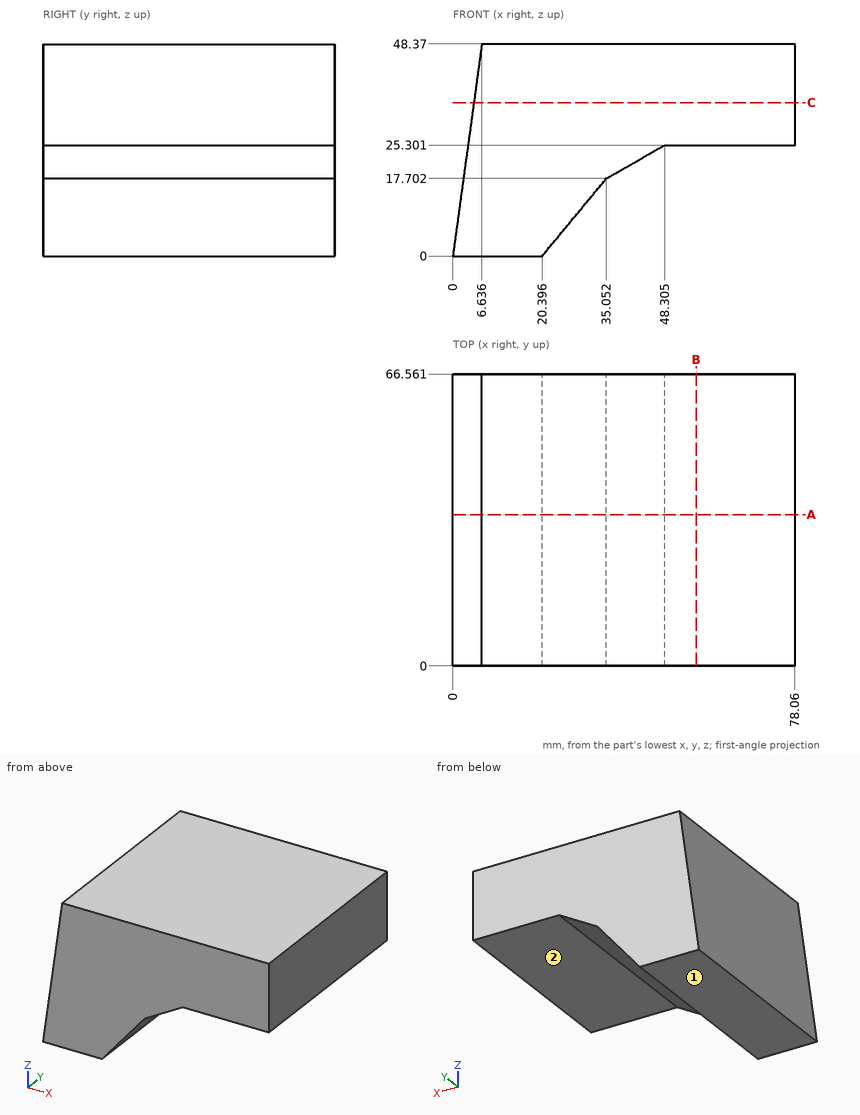
Geometry check sheet. Reference: drawing and pictorial views, mm from the part's lowest x, y, z. A direction names the side the tool comes from. Coordinates: 2 decimals unless noted, no trailing zeros. Loops run counter-clockwise (first coordinate to the right, second up) from the corner with the lowest first, then second, coordinate; pieces in that order, holes last. Notation, with made-up numbers: (44.5, 23) -> (96.5, 23) arc R18 cw to (96.5, 46) -> close; hole circle Ø4 at (77, 5). An arc over 180 degrees is marked (long way). Write item = value, one per line. Start each with the question number.
1. Material ranges on line 1 (Z direction, x = 60, y = 57); line 2 (Z direction, x = 32, y = 7) (1 decimal); line 3 (X direction, y = 16, z = 2) (1 decimal), recorded low to high.
2. Depth check by flat-ended pin: P1, Ø4, axis at x = 51.5, y = 34, coming from the -Z side; P2, Ø1.5, axis at x = 35.5, y = 59, coming from the -Z side; P3, Ø2, axis at y = 15, z = 5, coming from the -X side. Enter the tip coordinate at first touch or a pass-through.
3. Section check B-B on x = 55.5. Record the cut outline in (y, z), then the cut area to 3 significant figures.
4. Section check C-C on z = 35. Record the cut outline in (x, y), then the cut area to 3 significant figures.
5. Section check A-A on y = 34.5. Record the cut outline in (x, z) (1 decimal), then the cut area to 3 significant figures.
6. Tool access check on the marked faces 1 and 2. Record the directions out of +Z, -Z, +X, -X, +Y, -Y that give a thin tool (end or side, any length) a straight path to the whole face; none if there is none.
Responses:
q1.line_1 = 25.3 to 48.37
q1.line_2 = 14 to 48.4
q1.line_3 = 0.3 to 22.1
q2.P1 = 25.3
q2.P2 = 17.34
q2.P3 = 0.55
q3.outline = (0, 25.3) -> (66.56, 25.3) -> (66.56, 48.37) -> (0, 48.37) -> close
q3.area = 1,540 mm2
q4.outline = (4.8, 0) -> (78.06, 0) -> (78.06, 66.56) -> (4.8, 66.56) -> close
q4.area = 4,880 mm2
q5.outline = (0, 0) -> (20.4, 0) -> (35.1, 17.7) -> (48.3, 25.3) -> (78.1, 25.3) -> (78.1, 48.4) -> (6.6, 48.4) -> close
q5.area = 2,450 mm2
q6.face_1 = -Z, +X, -X, +Y, -Y
q6.face_2 = -Z, +X, +Y, -Y
